Input: part model. Units: mm. Frame: model coordinates. Coordinates: 2 decimals unless noted, no trailing zeros. Order: outer loops, then holes, each group sorted by start corner. A loop starts at its lowest first (then second) coordinate and runs counter-clockwise, first axis right, second up.
from build123d import *

# Parameters (mm, degrees)
SKETCH1_R           = 49.5046
BOSS_EXTRUDE1_DEPTH = 5.08
SKETCH2_R           = 47.625
BOSS_EXTRUDE2_DEPTH = 3.175
SKETCH3_R           = 6.731
SKETCH3_R_2         = 3.96875
SKETCH3_R_3         = 9.525
CUT_EXTRUDE1_DEPTH  = 9.255
SKETCH4_R           = 55.708104083
CUT_EXTRUDE2_DEPTH  = 3.175


with BuildPart() as part:
    # Sketch1 → Boss-Extrude1 (new body)
    with BuildSketch(Plane.XY):
        Circle(SKETCH1_R)
    extrude(amount=BOSS_EXTRUDE1_DEPTH)

    # Sketch2 → Boss-Extrude2 (add)
    with BuildSketch(Plane.XY.offset(5.08)):
        Circle(SKETCH2_R)
    extrude(amount=BOSS_EXTRUDE2_DEPTH)

    # Sketch3 → Cut-Extrude1 (cut, through all)
    with BuildSketch(Plane.XY.offset(8.255)):
        with Locations((-12.7, -31.166793627)):
            Circle(SKETCH3_R)
        with Locations((12.7, -31.166793627)):
            Circle(SKETCH3_R)
        with Locations((-36.83, 0)):
            Circle(SKETCH3_R_2)
        with Locations((36.83, 0)):
            Circle(SKETCH3_R_2)
        Circle(SKETCH3_R_3)
    extrude(amount=-CUT_EXTRUDE1_DEPTH, mode=Mode.SUBTRACT)

    # Sketch4 → Cut-Extrude2 (cut)
    with BuildSketch(Plane.XY.offset(8.255)):
        Circle(SKETCH4_R)
    extrude(amount=-CUT_EXTRUDE2_DEPTH, mode=Mode.SUBTRACT)


solid = part.part
Item 1: Ray query, probe 1 along X at (y, z) = (-2, 2.9); probe 2 along Y at (x, z) = (7, 2.9); probe 3 along X at (y, z) = (-29.5, 4.85). Return the intervals inside material, ascending.
Response values:
probe 1: x = -49.46 to -40.26, -33.4 to -9.31, 9.31 to 33.4, 40.26 to 49.46
probe 2: y = -49.01 to -34.75, -27.59 to -6.46, 6.46 to 49.01
probe 3: x = -39.75 to -19.22, -6.18 to 6.18, 19.22 to 39.75
Item 2: Cut plane B-B on y = -29. Return loops of the section in (x, z), then the cut area to 3 significant figures.
Response values:
outline: (-40.12, 0) - (-19.07, 0) - (-19.07, 5.08) - (-40.12, 5.08) - close; (-6.33, 0) - (6.33, 0) - (6.33, 5.08) - (-6.33, 5.08) - close; (19.07, 0) - (40.12, 0) - (40.12, 5.08) - (19.07, 5.08) - close
area: 278 mm2
Item 3: Cut plane D-D on x = -35. Return loops of the section in (y, z).
Response values:
outline: (-35.01, 0) - (-3.52, 0) - (-3.52, 5.08) - (-35.01, 5.08) - close; (3.52, 0) - (35.01, 0) - (35.01, 5.08) - (3.52, 5.08) - close
Item 4: Cut plane C-C on z = 3.55. Count the separate pieces of the cut face and the enclosed holes in it, then the cut area to 3 significant figures.
Response values:
separate pieces: 1
enclosed holes: 5
area: 7,030 mm2
Item 5: Draft query along X for faces 1 (the face through (-13.576, -24.493, 2.576)), 2 (the face through (-6.445, 49.083, 2.504)), 3 (the face through (10, 1, 5.08)). Return one class per face: pulls with the +X half, pulls with the -X half, needs draft (parallel to the pull), parting line crosses it, or undercut.
Response values:
face 1: undercut
face 2: parting line crosses it
face 3: needs draft
Item 6: Pin query (flat end, axial travel): pin 1 Ø11 at (x, y) = (-12.7, -31.17) entering from -Z; pin 2 Ø1.5 at (x, y) = (3.5, 36.5) entering from -Z; pin 3 Ø1.5 at (y, z) = (-5.5, 4) entering from +X; pin 4 Ø1 at (x, z) = (13, 2) entering from +Y. Return the tip coordinate at first contact, or that it passes through.
Response values:
pin 1: passes through
pin 2: stops at z = 0
pin 3: stops at x = 49.28
pin 4: stops at y = 47.9
Item 7: Cut plane A-A on x = 0. Return loops of the section in (y, z) (3 decimals), then the cut area to 3 significant figures.
Response values:
outline: (-49.505, 0) - (-9.525, 0) - (-9.525, 5.08) - (-49.505, 5.08) - close; (9.525, 0) - (49.505, 0) - (49.505, 5.08) - (9.525, 5.08) - close
area: 406 mm2
